Check sheet for the modelled part. Datum: model origin and axes. Units: mm. A direction names the side the tool comes from. Give positions to 0.01 mm unless a question says otherwise; leave off trailing zeros. Order: outer loops, then holes, each group sorted by start corner. A loop starts at its lowest first (then second) coordinate and runs counter-clockwise, first axis right, second up.
from build123d import *

# Parameters (mm, degrees)
ESQUISSE1_R        = 2.15
BOSS_EXTRU_1_DEPTH = 50


with BuildPart() as part:
    # Esquisse1 → Boss.-Extru.1 (new body)
    with BuildSketch(Plane(origin=(0, 0, 0), x_dir=(-1, 0, 0), z_dir=(0, 0, -1))):
        with BuildLine():
            Line((-40, 6.7), (-40, 2))
            ThreePointArc((-40, 2), (-39.414213562, 0.585786438), (-38, 0))
            Line((-38, 0), (-33.3, 0))
            ThreePointArc((-33.3, 0), (-32.734314575, 0.234314575), (-32.5, 0.8))
            Line((-32.5, 0.8), (-32.5, 1.5))
            ThreePointArc((-32.5, 1.5), (-32.587867966, 1.712132034), (-32.8, 1.8))
            Line((-32.8, 1.8), (-34.918424061, 1.8))
            ThreePointArc((-34.918424061, 1.8), (-35.686700051, 2.313345604), (-35.506437047, 3.219588924))
            Line((-35.506437047, 3.219588924), (-33.254705627, 5.471320344))
            ThreePointArc((-33.254705627, 5.471320344), (-32.281435581, 6.121638598), (-31.133385284, 6.35))
            Line((-31.133385284, 6.35), (-28.866614716, 6.35))
            ThreePointArc((-28.866614716, 6.35), (-27.718564419, 6.121638598), (-26.745294373, 5.471320344))
            Line((-26.745294373, 5.471320344), (-24.493562953, 3.219588924))
            ThreePointArc((-24.493562953, 3.219588924), (-24.313299949, 2.313345604), (-25.081575939, 1.8))
            Line((-25.081575939, 1.8), (-27.2, 1.8))
            ThreePointArc((-27.2, 1.8), (-27.412132034, 1.712132034), (-27.5, 1.5))
            Line((-27.5, 1.5), (-27.5, 0.8))
            ThreePointArc((-27.5, 0.8), (-27.265685425, 0.234314575), (-26.7, 0))
            Line((-26.7, 0), (-13.3, 0))
            ThreePointArc((-13.3, 0), (-12.734314575, 0.234314575), (-12.5, 0.8))
            Line((-12.5, 0.8), (-12.5, 1.5))
            ThreePointArc((-12.5, 1.5), (-12.587867966, 1.712132034), (-12.8, 1.8))
            Line((-12.8, 1.8), (-14.918424061, 1.8))
            ThreePointArc((-14.918424061, 1.8), (-15.686700051, 2.313345604), (-15.506437047, 3.219588924))
            Line((-15.506437047, 3.219588924), (-13.254705627, 5.471320344))
            ThreePointArc((-13.254705627, 5.471320344), (-12.281435581, 6.121638598), (-11.133385284, 6.35))
            Line((-11.133385284, 6.35), (-8.866614716, 6.35))
            ThreePointArc((-8.866614716, 6.35), (-7.718564419, 6.121638598), (-6.745294373, 5.471320344))
            Line((-6.745294373, 5.471320344), (-4.493562953, 3.219588924))
            ThreePointArc((-4.493562953, 3.219588924), (-4.313299949, 2.313345604), (-5.081575939, 1.8))
            Line((-5.081575939, 1.8), (-7.2, 1.8))
            ThreePointArc((-7.2, 1.8), (-7.412132034, 1.712132034), (-7.5, 1.5))
            Line((-7.5, 1.5), (-7.5, 0.8))
            ThreePointArc((-7.5, 0.8), (-7.265685425, 0.234314575), (-6.7, 0))
            Line((-6.7, 0), (-2, 0))
            ThreePointArc((-2, 0), (-0.585786438, 0.585786438), (0, 2))
            Line((0, 2), (0, 6.7))
            ThreePointArc((0, 6.7), (-0.234314575, 7.265685425), (-0.8, 7.5))
            Line((-0.8, 7.5), (-1.5, 7.5))
            ThreePointArc((-1.5, 7.5), (-1.712132034, 7.412132034), (-1.8, 7.2))
            Line((-1.8, 7.2), (-1.8, 5.081575939))
            ThreePointArc((-1.8, 5.081575939), (-2.313345604, 4.313299949), (-3.219588924, 4.493562953))
            Line((-3.219588924, 4.493562953), (-5.471320344, 6.745294373))
            ThreePointArc((-5.471320344, 6.745294373), (-6.121638598, 7.718564419), (-6.35, 8.866614716))
            Line((-6.35, 8.866614716), (-6.35, 11.133385284))
            ThreePointArc((-6.35, 11.133385284), (-6.121638598, 12.281435581), (-5.471320344, 13.254705627))
            Line((-5.471320344, 13.254705627), (-3.219588924, 15.506437047))
            ThreePointArc((-3.219588924, 15.506437047), (-2.313345604, 15.686700051), (-1.8, 14.918424061))
            Line((-1.8, 14.918424061), (-1.8, 12.8))
            ThreePointArc((-1.8, 12.8), (-1.712132034, 12.587867966), (-1.5, 12.5))
            Line((-1.5, 12.5), (-0.8, 12.5))
            ThreePointArc((-0.8, 12.5), (-0.234314575, 12.734314575), (0, 13.3))
            Line((0, 13.3), (0, 18))
            ThreePointArc((0, 18), (-0.585786438, 19.414213562), (-2, 20))
            Line((-2, 20), (-6.7, 20))
            ThreePointArc((-6.7, 20), (-7.265685425, 19.765685425), (-7.5, 19.2))
            Line((-7.5, 19.2), (-7.5, 18.5))
            ThreePointArc((-7.5, 18.5), (-7.412132034, 18.287867966), (-7.2, 18.2))
            Line((-7.2, 18.2), (-5.081575939, 18.2))
            ThreePointArc((-5.081575939, 18.2), (-4.313299949, 17.686654396), (-4.493562953, 16.780411076))
            Line((-4.493562953, 16.780411076), (-6.745294373, 14.528679656))
            ThreePointArc((-6.745294373, 14.528679656), (-7.718564419, 13.878361402), (-8.866614716, 13.65))
            Line((-8.866614716, 13.65), (-11.133385284, 13.65))
            ThreePointArc((-11.133385284, 13.65), (-12.281435581, 13.878361402), (-13.254705627, 14.528679656))
            Line((-13.254705627, 14.528679656), (-15.506437047, 16.780411076))
            ThreePointArc((-15.506437047, 16.780411076), (-15.686700051, 17.686654396), (-14.918424061, 18.2))
            Line((-14.918424061, 18.2), (-12.8, 18.2))
            ThreePointArc((-12.8, 18.2), (-12.587867966, 18.287867966), (-12.5, 18.5))
            Line((-12.5, 18.5), (-12.5, 19.2))
            ThreePointArc((-12.5, 19.2), (-12.734314575, 19.765685425), (-13.3, 20))
            Line((-13.3, 20), (-26.7, 20))
            ThreePointArc((-26.7, 20), (-27.265685425, 19.765685425), (-27.5, 19.2))
            Line((-27.5, 19.2), (-27.5, 18.5))
            ThreePointArc((-27.5, 18.5), (-27.412132034, 18.287867966), (-27.2, 18.2))
            Line((-27.2, 18.2), (-25.081575939, 18.2))
            ThreePointArc((-25.081575939, 18.2), (-24.313299949, 17.686654396), (-24.493562953, 16.780411076))
            Line((-24.493562953, 16.780411076), (-26.745294373, 14.528679656))
            ThreePointArc((-26.745294373, 14.528679656), (-27.718564419, 13.878361402), (-28.866614716, 13.65))
            Line((-28.866614716, 13.65), (-31.133385284, 13.65))
            ThreePointArc((-31.133385284, 13.65), (-32.281435581, 13.878361402), (-33.254705627, 14.528679656))
            Line((-33.254705627, 14.528679656), (-35.506437047, 16.780411076))
            ThreePointArc((-35.506437047, 16.780411076), (-35.686700051, 17.686654396), (-34.918424061, 18.2))
            Line((-34.918424061, 18.2), (-32.8, 18.2))
            ThreePointArc((-32.8, 18.2), (-32.587867966, 18.287867966), (-32.5, 18.5))
            Line((-32.5, 18.5), (-32.5, 19.2))
            ThreePointArc((-32.5, 19.2), (-32.734314575, 19.765685425), (-33.3, 20))
            Line((-33.3, 20), (-38, 20))
            ThreePointArc((-38, 20), (-39.414213562, 19.414213562), (-40, 18))
            Line((-40, 18), (-40, 13.3))
            ThreePointArc((-40, 13.3), (-39.765685425, 12.734314575), (-39.2, 12.5))
            Line((-39.2, 12.5), (-38.5, 12.5))
            ThreePointArc((-38.5, 12.5), (-38.287867966, 12.587867966), (-38.2, 12.8))
            Line((-38.2, 12.8), (-38.2, 14.918424061))
            ThreePointArc((-38.2, 14.918424061), (-37.686654396, 15.686700051), (-36.780411076, 15.506437047))
            Line((-36.780411076, 15.506437047), (-34.528679656, 13.254705627))
            ThreePointArc((-34.528679656, 13.254705627), (-33.878361402, 12.281435581), (-33.65, 11.133385284))
            Line((-33.65, 11.133385284), (-33.65, 8.866614716))
            ThreePointArc((-33.65, 8.866614716), (-33.878361402, 7.718564419), (-34.528679656, 6.745294373))
            Line((-34.528679656, 6.745294373), (-36.780411076, 4.493562953))
            ThreePointArc((-36.780411076, 4.493562953), (-37.686654396, 4.313299949), (-38.2, 5.081575939))
            Line((-38.2, 5.081575939), (-38.2, 7.2))
            ThreePointArc((-38.2, 7.2), (-38.287867966, 7.412132034), (-38.5, 7.5))
            Line((-38.5, 7.5), (-39.2, 7.5))
            ThreePointArc((-39.2, 7.5), (-39.765685425, 7.265685425), (-40, 6.7))
        make_face()
        with Locations(Location((-10, 10, 0), (0, 0, 180))):
            Circle(ESQUISSE1_R, mode=Mode.SUBTRACT)
        with Locations(Location((-30, 10, 0), (0, 0, 180))):
            Circle(ESQUISSE1_R, mode=Mode.SUBTRACT)
        with BuildLine():
            Line((-18.585786174, 17.312993861), (-14.528681072, 13.255889759))
            ThreePointArc((-14.528681072, 13.255889759), (-13.878362627, 12.282619622), (-13.650001154, 11.134569154))
            Line((-13.650001154, 11.134569154), (-13.650001154, 8.865431094))
            ThreePointArc((-13.650001154, 8.865431094), (-13.878362476, 7.717381202), (-14.5286805, 6.7441115))
            Line((-14.5286805, 6.7441115), (-18.585786, 2.687006))
            ThreePointArc((-18.585786, 2.687006), (-19.999999562, 2.101219562), (-21.414213125, 2.687006))
            Line((-21.414213125, 2.687006), (-25.471320125, 6.744113))
            ThreePointArc((-25.471320125, 6.744113), (-26.121638379, 7.717383046), (-26.349999781, 8.865433344))
            Line((-26.349999781, 8.865433344), (-26.349999781, 11.134567344))
            ThreePointArc((-26.349999781, 11.134567344), (-26.121638308, 12.282617811), (-25.471319863, 13.255887949))
            Line((-25.471319863, 13.255887949), (-21.41421295, 17.312993861))
            ThreePointArc((-21.41421295, 17.312993861), (-19.999999562, 17.898780125), (-18.585786174, 17.312993861))
        make_face(mode=Mode.SUBTRACT)
    extrude(amount=-BOSS_EXTRU_1_DEPTH)


solid = part.part
1) Section check D-D, the plane x = 10.5. Record the cut outline in (y, z), then the cut area to 3 significant figures.
Recorded:
outline: (6.35, 0) - (7.91, 0) - (7.91, 50) - (6.35, 50) - close; (12.09, 0) - (13.65, 0) - (13.65, 50) - (12.09, 50) - close
area: 156 mm2
2) Draft check along X on faces 4 (the face through (36, 20, 25)), 5 (the face through (40, 16, 25)), 6 (the face through (7.703, 13.885, 24.65)), 7 (the face through (34.396, 4.33, 24.65)). Enter one of: +X half, -X half, draft (parallel to the pull), parting line (faces both ways), or undercut.
Recorded:
face 4: draft
face 5: +X half
face 6: undercut
face 7: undercut
3) Material ranges on L1, parallel to X at y = 10, z = 36; L2, parallel to Y at x = 30, z = 26; L3, parallel to Y at x = 14.5, z = 16, recorded low to high.
Recorded:
L1: x = 6.35 to 7.85, 12.15 to 13.65, 26.35 to 27.85, 32.15 to 33.65
L2: y = 6.35 to 7.85, 12.15 to 13.65
L3: y = 0 to 1.8, 4.23 to 6.77, 13.23 to 15.77, 18.2 to 20
4) Section check C-C, the plane z = 40.5. State how many separate pieces and enclosed holes the cut face has, then the cut area to 3 significant figures.
Recorded:
separate pieces: 1
enclosed holes: 3
area: 332 mm2
5) Depth check by flat-ended pin: pin 1 Ø0.6 at (y, z) = (1, 30) entering from -X; pin 2 Ø2.5 at (y, z) = (9.5, 31.5) entering from -X; pin 3 Ø0.8 at (y, z) = (19, 27) entering from +X; pin 4 Ø1.5 at (x, y) = (33.5, 17) entering from -Z. Enter the tip coordinate at first touch or a pass-through.
Recorded:
pin 1: stops at x = 0.13
pin 2: stops at x = 6.29
pin 3: stops at x = 39.91
pin 4: passes through
6) Section check A-A, the plane x = 30. Record the cut outline in (y, z), then the cut area to 3 significant figures.
Recorded:
outline: (6.35, 0) - (7.85, 0) - (7.85, 50) - (6.35, 50) - close; (12.15, 0) - (13.65, 0) - (13.65, 50) - (12.15, 50) - close
area: 150 mm2
7) Section check B-B, the plane y = 10. Record the cut outline in (x, z), then the cut area to 3 significant figures.
Recorded:
outline: (6.35, 0) - (7.85, 0) - (7.85, 50) - (6.35, 50) - close; (12.15, 0) - (13.65, 0) - (13.65, 50) - (12.15, 50) - close; (26.35, 0) - (27.85, 0) - (27.85, 50) - (26.35, 50) - close; (32.15, 0) - (33.65, 0) - (33.65, 50) - (32.15, 50) - close
area: 300 mm2
8) Set-up check for faces 1 (the face through (33.65, 10, 25)), 2 (the face through (35.67, 14.396, 24.65)), 3 (the face through (30, 13.65, 25)): record each of +Z, -Z, +X, -X, +Y, -Y from which the full face is reachable in a straight line by a thin tool's end or side.
Recorded:
face 1: +Z, -Z, +X
face 2: +Z, -Z
face 3: +Z, -Z, +Y
